Can you work these out from the model? Positions are in its coordinate system, mm. Face numbers are marked on the shaded views. A direction names the side the tool comes from. Round coordinates to 2 decimals unless told otherwise and drop trailing zeros. Order: outer loops, then holes, each group sorted by start corner. A loop starts at its lowest first (then second) coordinate and runs counter-clockwise, first axis right, second up.
Q1. If we section it at C-C (z = -19): Please give me the cut outline in (x, y).
Q2. If we section it at A-A (z = -47.5): Please give me the cut outline in (x, y).
Q3. If we section it at B-B (z = 18): Please give me the cut outline in (x, y).
Q4. Will these pins go through, and if not, where does the flat tip stop? P1, Ø3, axis at x = -16, z = -12, coming from the -Y side; P2, Ø5, axis at x = -19.5, y = -4, coming from the +Z side; P3, Ø1, axis at x = -19.5, y = -12.5, coming from the +Z side; P4, Ø9, axis at x = 0, z = -47.5, coming from the +Y side.
Q5. If I drill on line 1 (X direction, y = 0.75, z = -47.5); line 2 (Z direction, x = 0, y = -5.5); line 3 (Z direction, x = 0, y = -10.5), over which ranges is the centre line in solid material (lowest first)?
Q6. We'd pull the mould along Z, two halves only. Please class the marked faces 4, 5, 6 and 7: pulls with the +Z half, pulls with the -Z half, needs draft (parallel to the pull), parting line crosses it, or undercut.
Q7. For the marked faces 1, 2 and 3, which set-ups out of +Z, -Z, +X, -X, +Y, -Y let a thin tool reach every point of the face, with its end or its side?
Autodesk Inventor part; units mm, degrees
ref_plane "РабПлоскость1" through (0, 0, 0) normal (0, 0, 1) x (1, 0, 0)
ref_plane "РабПлоскость2" through (0, 0, -15) normal (0, 0, -1) x (-1, 0, 0)
ref_plane "РабПлоскость3" through (0, 0, -35) normal (0, 0, -1) x (-1, 0, 0)
sketch "Эскиз1" plane through (0, 0, 0) normal (0, 0, 1) x (1, 0, 0)
  circle A0 centre (0, 0) radius 9
sketch "Эскиз2" plane through (0, 0, 0) normal (0, 0, 1) x (1, 0, 0)
  point P0 (0, 0)
extrude "Выдавливание1" add sketch "Эскиз1" along normal blind 30
ref_plane "РабПлоскость1" through (0, 0, 0) normal (0, 0, 1) x (1, 0, 0)
sketch "Эскиз3" plane through (0, 0, 0) normal (0, 0, 1) x (1, 0, 0)
  circle A0 centre (0, 0) radius 25
extrude "Выдавливание2" add sketch "Эскиз3" against normal blind 15
ref_plane "РабПлоскость2" through (0, 0, -15) normal (0, 0, -1) x (-1, 0, 0)
sketch "Эскиз4" plane through (0, 0, -15) normal (0, 0, -1) x (-1, 0, 0)
  circle A0 centre (0, 0) radius 15
extrude "Выдавливание3" add sketch "Эскиз4" along normal blind 20
ref_plane "РабПлоскость3" through (0, 0, -35) normal (0, 0, -1) x (-1, 0, 0)
sketch "Эскиз5" plane through (0, 0, -35) normal (0, 0, -1) x (-1, 0, 0)
  circle A0 centre (0, 0) radius 15
extrude "Выдавливание4" add sketch "Эскиз5" along normal blind 25
ref_plane "РабПлоскость4" through (0, 0, -60) normal (0, 0, -1) x (-1, 0, 0)
sketch "Эскиз6" plane through (0, 0, -60) normal (0, 0, -1) x (-1, 0, 0)
  circle A0 centre (0, 0) radius 9
  circle A1 centre (0, 0) radius 15
extrude "Выдавливание5" add sketch "Эскиз6" along normal blind 20 contours A0 | A1
ref_plane "РабПлоскость5" through (0, 0, -80) normal (0, 0, -1) x (-1, 0, 0)
sketch "Эскиз7" plane through (0, 0, -80) normal (0, 0, -1) x (-1, 0, 0)
  circle A0 centre (0, 0) radius 15
  line L0 (0, 15) -> (15, 0)
  line L1 (15, 0) -> (0, -15)
  line L2 (0, -15) -> (-15, 0)
  line L3 (-15, 0) -> (0, 15)
extrude "Выдавливание6" add sketch "Эскиз7" along normal blind 20 contours L1 L2 L3 L0
sketch "Эскиз8" plane through (0, 0, 0) normal (1, 0, 0) x (0, 1, 0)
  line L0 (0, 0) -> (0, -35)
  line L1 (0, -35) -> (10, -35)
  line L2 (10, -35) -> (-10, -35)
  line L3 (-10, -35) -> (-10, -60)
  line L4 (-10, -60) -> (-25, -60)
  line L5 (-25, -60) -> (-25, -35)
  line L6 (-25, -35) -> (-10, -35)
  line L7 (10, -35) -> (10, -60)
  line L8 (10, -60) -> (25, -60)
  line L9 (25, -60) -> (25, -35)
  line L10 (25, -35) -> (10, -35)
  dimension "d22" = 35
  dimension "d23" = 10
  dimension "d24" = 20
  dimension "d25" = 25
  dimension "d26" = 15
  dimension "d27" = 15
extrude "Выдавливание7" cut sketch "Эскиз8" against normal mid plane 40 contours L10 L9 L8 L7
sketch "Эскиз9" plane through (0, 0, 0) normal (1, 0, 0) x (0, 1, 0)
  line L0 (0, 0) -> (0, -35)
  line L1 (0, -35) -> (-10, -35)
  line L2 (-10, -35) -> (-10, -60)
  line L3 (-10, -60) -> (-25, -60)
  line L4 (-25, -60) -> (-25, -35)
  line L5 (-25, -35) -> (-10, -35)
  dimension "d30" = 35
  dimension "d31" = 10
  dimension "d32" = 25
  dimension "d33" = 15
extrude "Выдавливание8" cut sketch "Эскиз9" along normal mid plane 40
sketch "Эскиз10" plane through (0, 0, 0) normal (1, 0, 0) x (0, 1, 0)
  point P0 (0, 0)
sketch "Эскиз11" plane through (0, 0, 0) normal (0, 1, 0) x (-1, 0, 0)
  line L0 (0, 0) -> (0, -47.5)
  circle A0 centre (0, -47.5) radius 5
  dimension "d36" = 47.5
  dimension "d37" = 10
extrude "Выдавливание9" cut sketch "Эскиз11" along normal mid plane 40
chamfer "Фаска1" distance 2.5 angle 45 1 edges at (-9, 0, 30)
chamfer "Фаска2" distance 10 angle 30 1 edges at (-25, 0, 0) measured on face at (19.3373, -2.7122, 0)
sketch "Эскиз12" plane through (0, 0, 0) normal (0, 1, 0) x (-1, 0, 0)
  line L0 (0, 0) -> (25, 0)
  line L1 (25, 0) -> (25, 4)
  line L2 (25, 4) -> (25, 6)
  line L3 (25, 6) -> (-25.3406, 6)
  line L4 (-25.3406, 6) -> (-25.3406, 0)
  line L5 (-25.3406, 0) -> (25, 0)
  dimension "d48" = 4
  dimension "d49" = 2
extrude "Выдавливание10" cut sketch "Эскиз12" against normal mid plane 40
sketch "Эскиз13" plane through (0, 0, 0) normal (0, 0, 1) x (1, 0, 0)
  circle A0 centre (0, 0) radius 7.25
  dimension "d52" = 14.5
extrude "Выдавливание11" add sketch "Эскиз13" along normal blind 6
fillet "Сопряжение1" radius 1 1 edges at (-7.25, 0, 6)
thread "Резьба2"
fillet "Сопряжение2" radius 1.6 1 edges at (-7.25, 0, 0)
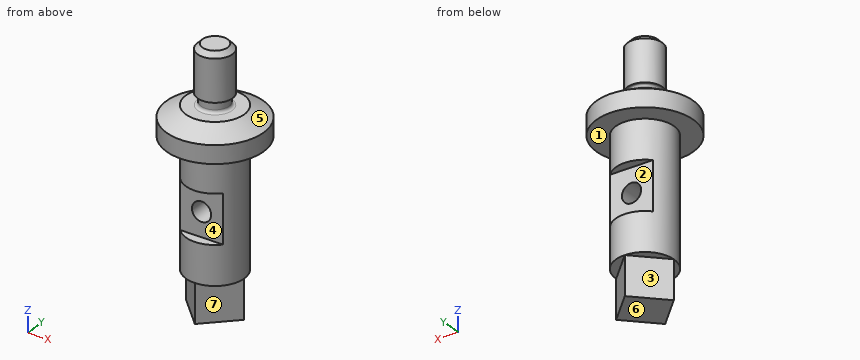
Solution:
1. outline: circle Ø30 at (0, 0)
2. outline: (-11.18, -10) - (-5, -10) - (-5, 10) - (-11.18, 10) arc R15 ccw to start; (5, -10) - (11.18, -10) arc R15 ccw to (11.18, 10) - (5, 10) - close
3. outline: circle Ø18 at (0, 0)
4. P1: stops at y = -20.37
4. P2: stops at z = -1.39
4. P3: stops at z = -4.42
4. P4: passes through
5. line 1: x = -14.98 to -5, 5 to 14.98
5. line 2: z = -100 to -52.5, -42.5 to 30
5. line 3: z = -100 to -60, -35 to 0
6. face 4: undercut
6. face 5: pulls with the +Z half
6. face 6: pulls with the -Z half
6. face 7: needs draft
7. face 1: -Z
7. face 2: +X, -X, +Y
7. face 3: -Z, -X, +Y
